Read the model definition and answer for the solid it produces. Units are mm, in the model's axes. Face numbers are marked on the shaded views. A direction names the side the tool comes from. Coordinates: 2 decimals unless noted, no trailing zeros. Loops run counter-clockwise (first coordinate to the right, second up) from the corner with the lowest first, then second, coordinate; pieces in that order, holes last.
Q1. Straight lines are drawn through the part: line 1 (Z direction, x = 6.5, y = 19.5); line 2 (X direction, y = -16.5, z = 3.5). For each, find the intervals that lie inside material, in ascending order.
Q2. Section D-D (x = -21) is taken. Give the vertices of the cut face in (y, z), then the cut area to 3 significant figures.
Q3. Section C-C (z = 23) is taken. Give the vertices of the cut face in (x, y), then the cut area to 3 significant figures.
Q4. Section A-A (x = 0) is taken. Give the vertices of the cut face in (y, z), then the cut area to 3 significant figures.
Q5. The mould has two halves that part along Y. Classify the marked faces 1, 2 and 3: pulls with the +Y half, pulls with the -Y half, needs draft (parallel to the pull), parting line crosses it, or undercut.
Q6. Which of the six approach directions +Z, -Z, +X, -X, +Y, -Y give full straight-line access (tool end or side, diameter ignored) to the marked faces 4 and 5?
Q7. Flat-ended cylindrical pins translate along their axes: P1, Ø2, axis at x = 36, y = -2, coming from the +Z side; P2, Ø3, axis at x = 8, y = -7.5, coming from the +Z side; P3, Ø1.3, axis at x = -35.5, z = 3.5, coming from the +Y side. Find the tip coordinate at first contact, or state that the pin passes through.
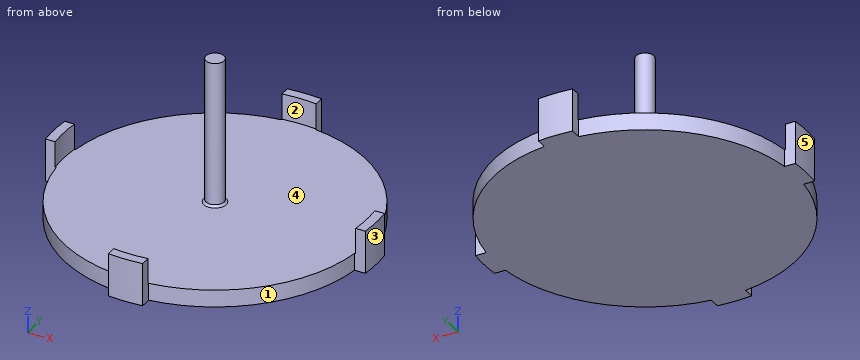
from build123d import *

# Parameters (mm, degrees)
BOSS_EXTRUDE1_DEPTH   = 10
BOSS_EXTRUDE1_2_DEPTH = 10
BOSS_EXTRUDE1_3_DEPTH = 10
BOSS_EXTRUDE1_4_DEPTH = 10
SKETCH1_3_R           = 35
BOSS_EXTRUDE2_DEPTH   = 4
SKETCH3_R             = 2.1
BOSS_EXTRUDE3_DEPTH   = 34
FILLET1_R             = 0.5


with BuildPart() as part:
    # Sketch1 → Boss-Extrude1 (new body)
    with BuildSketch(Plane.XY):
        with BuildLine():
            ThreePointArc((-35.022314315, -4), (-35.25, 0), (-35.022314315, 4))
            Line((-35.022314315, 4), (-37.286056375, 4))
            ThreePointArc((-37.286056375, 4), (-37.5, 0), (-37.286056375, -4))
            Line((-37.286056375, -4), (-35.022314315, -4))
        make_face()
    extrude(amount=BOSS_EXTRUDE1_DEPTH)



with BuildPart() as body_2:
    # Sketch1 → Boss-Extrude1 2 (new body)
    with BuildSketch(Plane.XY):
        with BuildLine():
            ThreePointArc((-4, 35.022314315), (0, 35.25), (4, 35.022314315))
            Line((4, 35.022314315), (4, 37.286056375))
            ThreePointArc((4, 37.286056375), (0, 37.5), (-4, 37.286056375))
            Line((-4, 37.286056375), (-4, 35.022314315))
        make_face()
    extrude(amount=BOSS_EXTRUDE1_2_DEPTH)


with BuildPart() as body_3:
    # Sketch1 → Boss-Extrude1 3 (new body)
    with BuildSketch(Plane.XY):
        with BuildLine():
            ThreePointArc((37.286056375, -4), (37.5, 0), (37.286056375, 4))
            Line((37.286056375, 4), (35.022314315, 4))
            ThreePointArc((35.022314315, 4), (35.25, 0), (35.022314315, -4))
            Line((35.022314315, -4), (37.286056375, -4))
        make_face()
    extrude(amount=BOSS_EXTRUDE1_3_DEPTH)


with BuildPart() as body_4:
    # Sketch1 → Boss-Extrude1 4 (new body)
    with BuildSketch(Plane.XY):
        with BuildLine():
            Line((4, -37.286056375), (4, -35.022314315))
            ThreePointArc((4, -35.022314315), (0, -35.25), (-4, -35.022314315))
            Line((-4, -35.022314315), (-4, -37.286056375))
            ThreePointArc((-4, -37.286056375), (0, -37.5), (4, -37.286056375))
        make_face()
    extrude(amount=BOSS_EXTRUDE1_4_DEPTH)


with BuildPart() as part_1:
    add(part.part)

    add(body_2.part)  # Boss-Extrude2 merges body 2

    add(body_3.part)  # Boss-Extrude2 merges body 3

    add(body_4.part)  # Boss-Extrude2 merges body 4
    # Sketch1_3 → Boss-Extrude2 (add)
    with BuildSketch(Plane.XY):
        Circle(SKETCH1_3_R)
        with BuildLine():
            ThreePointArc((-34.770677301, -4), (-35, 0), (-34.770677301, 4))
            Line((-34.770677301, 4), (-35.022314315, 4))
            ThreePointArc((-35.022314315, 4), (-35.25, 0), (-35.022314315, -4))
            Line((-35.022314315, -4), (-34.770677301, -4))
        make_face()
        with BuildLine():
            Line((4, -35.022314315), (4, -34.770677301))
            ThreePointArc((4, -34.770677301), (0, -35), (-4, -34.770677301))
            Line((-4, -34.770677301), (-4, -35.022314315))
            ThreePointArc((-4, -35.022314315), (0, -35.25), (4, -35.022314315))
        make_face()
        with BuildLine():
            ThreePointArc((-4, 34.770677301), (0, 35), (4, 34.770677301))
            Line((4, 34.770677301), (4, 35.022314315))
            ThreePointArc((4, 35.022314315), (0, 35.25), (-4, 35.022314315))
            Line((-4, 35.022314315), (-4, 34.770677301))
        make_face()
        with BuildLine():
            ThreePointArc((35.022314315, -4), (35.25, 0), (35.022314315, 4))
            Line((35.022314315, 4), (34.770677301, 4))
            ThreePointArc((34.770677301, 4), (34.942622294, 2.00328411), (35, 0))
            ThreePointArc((35, 0), (34.942622294, -2.00328411), (34.770677301, -4))
            Line((34.770677301, -4), (35.022314315, -4))
        make_face()
    extrude(amount=BOSS_EXTRUDE2_DEPTH)

    # Sketch3 → Boss-Extrude3 (add)
    with BuildSketch(Plane.XY.offset(4)):
        Circle(SKETCH3_R)
    extrude(amount=BOSS_EXTRUDE3_DEPTH)

    # Fillet1
    fillet1_edges = [part_1.edges().sort_by_distance(p)[0] for p in [
        (-2.1, 0, 4),
    ]]
    fillet(fillet1_edges, radius=FILLET1_R)


solid = part_1.part
Numbers:
1. line 1: z = 0 to 4
1. line 2: x = -30.87 to 30.87
2. outline: (-28, 0) - (28, 0) - (28, 4) - (-28, 4) - close
2. area: 224 mm2
3. outline: circle Ø4.2 at (0, 0)
3. area: 13.9 mm2
4. outline: (-37.5, 0) - (37.5, 0) - (37.5, 10) - (35.25, 10) - (35.25, 4) - (2.6, 4) arc R0.5 cw to (2.1, 4.5) - (2.1, 38) - (-2.1, 38) - (-2.1, 4.5) arc R0.5 cw to (-2.6, 4) - (-35.25, 4) - (-35.25, 10) - (-37.5, 10) - close
4. area: 470 mm2
5. face 1: pulls with the -Y half
5. face 2: undercut
5. face 3: parting line crosses it
6. face 4: +Z
6. face 5: +Z, -Z, -X
7. P1: stops at z = 10
7. P2: stops at z = 4
7. P3: stops at y = 4
